```python
from build123d import *

# Parameters (mm, degrees)
F0_R        = 10
F1_DEPTH    = 25
F2_DEPTH    = 50
F3_SIZE     = 2
F4_T4_DEPTH = 123.4369555733
F4_S5_R     = 25
F4_T6_DEPTH = 64


# Not quite as in the source:
# - a fillet or chamfer that OpenCascade refuses, or shapes differently, is made with other operations: its cross-section is extruded or revolved along the edge and cut away or added


with BuildPart() as f1:
    # F0 (on Front) → F1 (new body)
    with BuildSketch(Plane.XZ):
        with BuildLine():
            ThreePointArc((2.0833333333, -24.9130432148), (18.3995018048, -16.9250800097), (25, 0))
            ThreePointArc((25, 0), (18.3995018048, 16.9250800097), (2.0833333333, 24.9130432148))
            ThreePointArc((2.0833333333, 24.9130432148), (-25, 0), (2.0833333333, -24.9130432148))
        make_face()
        Circle(F0_R, mode=Mode.SUBTRACT)
        with BuildLine():
            ThreePointArc((2.0833333333, 24.9130432148), (18.3995018048, 16.9250800097), (25, 0))
            ThreePointArc((25, 0), (18.3995018048, -16.9250800097), (2.0833333333, -24.9130432148))
            Line((2.0833333333, -24.9130432148), (91.4583333333, -17.4391302504))
            ThreePointArc((91.4583333333, -17.4391302504), (72.5, 0), (91.4583333333, 17.4391302504))
            Line((91.4583333333, 17.4391302504), (2.0833333333, 24.9130432148))
        make_face()
        with BuildLine():
            ThreePointArc((107.5, 0), (102.8796512634, 11.8475560068), (91.4583333333, 17.4391302504))
            ThreePointArc((91.4583333333, 17.4391302504), (72.5, 0), (91.4583333333, -17.4391302504))
            ThreePointArc((91.4583333333, -17.4391302504), (102.8796512634, -11.8475560068), (107.5, 0))
        make_face()
        with Locations((90, 0)):
            Circle(F0_R, mode=Mode.SUBTRACT)
    extrude(amount=F1_DEPTH)

    # F0 (on Front) → F2 (join)
    with BuildSketch(Plane.XZ):
        with BuildLine():
            ThreePointArc((2.0833333333, -24.9130432148), (18.3995018048, -16.9250800097), (25, 0))
            ThreePointArc((25, 0), (18.3995018048, 16.9250800097), (2.0833333333, 24.9130432148))
            ThreePointArc((2.0833333333, 24.9130432148), (-25, 0), (2.0833333333, -24.9130432148))
        make_face()
        Circle(F0_R, mode=Mode.SUBTRACT)
    extrude(amount=F2_DEPTH)

    # F3
    f3_edges = [f1.edges().sort_by_distance(p)[0] for p in [
        (-2.083333, -50, 24.913043),
        (-10, -50, 0),
        (80, -25, 0),
    ]]
    chamfer(f3_edges, length=F3_SIZE)

    # F4: fillet of radius 5 on 1 edges, made by hand


with BuildPart() as f4_tool2:
    # F4_s3 → F4_t4 (new body)
    with BuildSketch(Plane(origin=(101.8315216074, 0, -8.5155796311), x_dir=(0, 1, 0), z_dir=(-0.9965217286, 0, 0.0833333333))):
        with BuildLine():
            ThreePointArc((-25, -20), (-23.5355339059, -23.5355339059), (-20, -25))
            Line((-20, -25), (-25, -25))
            Line((-25, -25), (-25, -20))
        make_face()
    extrude(amount=F4_T4_DEPTH)

    # F4_s5 → F4_t6 (cut, symmetric)
    with BuildSketch(Plane.XZ.offset(22.5)):
        Circle(F4_S5_R)
    extrude(amount=F4_T6_DEPTH, both=True, mode=Mode.SUBTRACT)


with BuildPart() as f1_1:
    add(f1.part)

    # F4_t1: cut F4_tool2
    add(f4_tool2.part, mode=Mode.SUBTRACT)


solid = f1_1.part
```
Check sheet for the modelled part. Datum: model origin and axes. Units: mm. Round coordinates to 2 decimals unless told otherwise and drop trailing zeros. Loops run counter-clockwise (first coordinate to the right, second up) from the corner with the lowest first, then second, coordinate; pieces in that order, holes last. Notation, with made-up numbers: (42, 33) - (69, 33) arc R13 ccw to (69, 55) - close; hole circle Ø9 at (59, 21.5). An arc over 180 degrees is marked (long way). Answer as a JSON object with one key per item and string values. Group by question number.
Q1. Gauge pin test, flat ends, axial feed: P1, Ø12, axis at y = -23.5, z = -9, coming from the -X side; P2, Ø6, axis at x = 51, y = -20, coming from the -Z side; P3, Ø12, axis at y = -34.5, z = -7.5, coming from the +X side. Record the tip position at first contact, or that the pin passes through.
Q2. Mould release check, pull along Z, two halves, no side actions. Record for faces 1 (the face through (47.396, -9.86, 21.124)), 2 (the face through (81.965, -23.125, -6.161)), 3 (the face through (40, 0, 0)): released by +Z, released by -Z, zero draft, split by the parting line, or undercut.
Q3. Sectioned sample at C-C, the plane y = -45.5. Enter the section's corners in (x, z), plus the area to 3 significant figures.
Q4. Scan lines: line 1 along Z through (x, y) = (0, -9.5); line 2 along Z through (x, y) = (-7, -25); line 3 along Y through (x, z) = (55.5, 12). Record each from-to range of solid material in increasing order. Write a range as [from, to].
Q5. Sectioned sample at A-A, the plane y = -15. Enter the section's corners in (x, z), plus the area to 3 significant figures.
Q6. Sectioned sample at B-B, the plane x = 0. Enter the section's corners in (y, z), plus the area to 3 significant figures.
Solution:
{
 "1": {"P1": "stops at x = -24.82", "P2": "stops at z = -21.07", "P3": "stops at x = 24.95"},
 "2": {"face 1": "released by +Z", "face 2": "undercut", "face 3": "zero draft"},
 "3": {"outline": "circle Ø50 at (0, 0); hole circle Ø20 at (0, 0)", "area": "1,650 mm²"},
 "4": {"line 1": "z = [-25, -10], [10, 25]", "line 2": "z = [-24, -7.14], [7.14, 24]", "line 3": "y = [-25, 0]"},
 "5": {"outline": "(2.08, -24.91) - (91.46, -17.44) arc R17.5 ccw to (91.46, 17.44) - (2.08, 24.91) arc R25 ccw (long way) to start; hole circle Ø20 at (0, 0); hole circle Ø20 at (90, 0)", "area": "4,670 mm²"},
 "6": {"outline": "(-50, -23) - (-48, -25) - (0, -25) - (0, -10) - (-48, -10) - (-50, -12) - close; (-50, 12) - (-48, 10) - (0, 10) - (0, 25) - (-48, 25) - (-50, 23) - close", "area": "1,490 mm²"}
}
